from build123d import *

# Parameters (mm, degrees)
ESQUISSE1_W             = 40
ESQUISSE1_H             = 70
BOSS_EXTRU_1_DEPTH      = 3
ESQUISSE4_W             = 40
ESQUISSE4_H             = 3
BOSS_EXTRU_3_DEPTH      = 143
ESQUISSE5_W             = 40
ESQUISSE5_H             = 30
BOSS_EXTRU_4_DEPTH      = 3
ESQUISSE6_R             = 4.5
ENL_V_MAT_EXTRU_1_DEPTH = 147
CONG_1_R                = 1
CONG_2_R                = 3
CONG_3_R                = 3
CONG_4_R                = 3
CONG_5_R                = 1


with BuildPart() as part:
    # Esquisse1 → Boss.-Extru.1 (new body)
    with BuildSketch(Plane.XY):
        Rectangle(ESQUISSE1_W, ESQUISSE1_H)
    extrude(amount=BOSS_EXTRU_1_DEPTH)

    # Esquisse4 → Boss.-Extru.3 (add)
    with BuildSketch(Plane.XY.offset(3)):
        with Locations((0, 36.5)):
            Rectangle(ESQUISSE4_W, ESQUISSE4_H)
        with Locations((0, -36.5)):
            Rectangle(ESQUISSE4_W, ESQUISSE4_H)
    extrude(amount=-BOSS_EXTRU_3_DEPTH)

    # Esquisse5 → Boss.-Extru.4 (add)
    with BuildSketch(Plane(origin=(0, 0, -140), x_dir=(-1, 0, 0), z_dir=(0, 0, -1))):
        with Locations((0, 50)):
            Rectangle(ESQUISSE5_W, ESQUISSE5_H)
        with Locations((0, -50)):
            Rectangle(ESQUISSE5_W, ESQUISSE5_H)
    extrude(amount=BOSS_EXTRU_4_DEPTH)

    # Esquisse6 → Enlèv. mat.-Extru.1 (cut, through all)
    with BuildSketch(Plane(origin=(0, 0, -143), x_dir=(-1, 0, 0), z_dir=(0, 0, -1))):
        with Locations((0, 50)):
            Circle(ESQUISSE6_R)
        with Locations((0, -50)):
            Circle(ESQUISSE6_R)
    extrude(amount=-ENL_V_MAT_EXTRU_1_DEPTH, mode=Mode.SUBTRACT)

    # Congé1
    cong_1_edges = [part.edges().sort_by_distance(p)[0] for p in [
        (0, 35, 0),
        (0, -35, 0),
    ]]
    fillet(cong_1_edges, radius=CONG_1_R)

    # Congé2
    cong_2_edges = [part.edges().sort_by_distance(p)[0] for p in [
        (0, 38, 3),
        (0, -38, 3),
    ]]
    fillet(cong_2_edges, radius=CONG_2_R)

    # Congé3
    cong_3_edges = [part.edges().sort_by_distance(p)[0] for p in [
        (0, 38, -140),
        (0, -38, -140),
    ]]
    fillet(cong_3_edges, radius=CONG_3_R)

    # Congé4
    cong_4_edges = [part.edges().sort_by_distance(p)[0] for p in [
        (0, 35, -143),
        (0, -35, -143),
    ]]
    fillet(cong_4_edges, radius=CONG_4_R)

    # Congé5
    cong_5_edges = [part.edges().sort_by_distance(p)[0] for p in [
        (4.5, 50, -140),
        (4.5, -50, -140),
    ]]
    fillet(cong_5_edges, radius=CONG_5_R)


solid = part.part
CAD build for the part. Positions are in the model's coordinates, mm. A direction names the side the tool comes from. Give positions to 0.01 mm unless a question says otherwise; leave off trailing zeros. Loops run counter-clockwise (first coordinate to the right, second up) from the corner with the lowest first, then second, coordinate; pieces in that order, holes last. Notation, with made-up numbers: M -8,-10 L 19,-10 A21 ccw 19,10 Z; hole C 2,1 d11. An arc over 180 degrees is marked long. Answer in a Markdown table with one row per item. Add a question column.
Item 1: Drop flat-ended pins along their axis: P1, Ø1, axis at x = 8.5, z = -42.5, coming from the +Y side; P2, Ø7, axis at x = 7.5, y = -51.5, coming from the +Z side; P3, Ø12, axis at x = -8, y = -12.5, coming from the -Z side. Give the stop position or say it passes through.
Item 2: Mould opens along X. For faces 1 (the face through (20, 0, 1)), 2 (the face through (0.98, -54.39, -142.01)), 3 (the face through (0, 0, 0)) say: +X half, -X half, draft (parallel to the pull), parting line (faces both ways), or undercut.
Item 3: Band-saw the part on B-B on z = -28. Give the cut face in (x, y).
Item 4: Tool access for faces 4 (the face through (0, -38, -68)), 5 (the face through (0, 35, -70)), 6 (the face through (0, 38, -68)), 7 (the face through (0, 65, -141)): list every direction of +Z, -Z, +X, -X, +Y, -Y with a clear straight run to the whole face (end or side of a thin tool).
Item 5: Band-saw the part on D-D on x = -11.5. Give the cut face in (y, z), then the cut area to 3 significant figures.
Item 6: Probe probe 1 along Y at (x, z) = (-18, -123.5); probe 2 along Y at (x, z) = (0, -142); probe 3 along Y at (x, z) = (0, -141.75). List the from-to ranges inside material, lowest first.
Item 7: Band-saw the part on C-C on y = -50. Give the cut face in (x, z).
Item 8: Band-saw the part on A-A on x = 0. Give the number of separate pieces and of enclosed holes in the cut face, then the cut area to 3 significant figures.
Reply:
| question | item | result |
|---|---|---|
| 1 | P1 | stops at y = 38 |
| 1 | P2 | stops at z = -140 |
| 1 | P3 | stops at z = 0 |
| 2 | face 1 | +X half |
| 2 | face 2 | undercut |
| 2 | face 3 | draft |
| 3 | outline | M -20,-38 L 20,-38 L 20,-35 L -20,-35 Z; M -20,35 L 20,35 L 20,38 L -20,38 Z |
| 4 | face 4 | +Z, +X, -X, -Y |
| 4 | face 5 | -Z, +X, -X |
| 4 | face 6 | +Z, +X, -X, +Y |
| 4 | face 7 | +Z, -Z, +X, -X, +Y |
| 5 | outline | M -65,-143 L -38,-143 A3 ccw -35,-140 L -35,-1 A1 cw -34,0 L 34,0 A1 cw 35,-1 L 35,-140 A3 ccw 38,-143 L 65,-143 L 65,-140 L 41,-140 A3 cw 38,-137 L 38,0 A3 ccw 35,3 L -35,3 A3 ccw -38,0 L -38,-137 A3 cw -41,-140 L -65,-140 Z |
| 5 | area | 1,240 mm^2 |
| 6 | probe 1 | y = -38 to -35, 35 to 38 |
| 6 | probe 2 | y = -65 to -54.5, -45.5 to -35.76, 35.76 to 45.5, 54.5 to 65 |
| 6 | probe 3 | y = -65 to -54.5, -45.5 to -35.56, 35.56 to 45.5, 54.5 to 65 |
| 7 | outline | M -20,-143 L -4.5,-143 L -4.5,-141 A1 ccw -5.5,-140 L -20,-140 Z; M 4.5,-143 L 20,-143 L 20,-140 L 5.5,-140 A1 ccw 4.5,-141 Z |
| 8 | separate pieces | 3 |
| 8 | enclosed holes | 0 |
| 8 | area | 1,190 mm^2 |
